from build123d import *

# Parameters (mm, degrees)
SKETCH1_R           = 3
BOSS_EXTRUDE1_DEPTH = 75
SKETCH2_R           = 5.8
BOSS_EXTRUDE2_DEPTH = 4.3
FILLET1_R           = 1


with BuildPart() as part:
    # Sketch1 → Boss-Extrude1 (new body)
    with BuildSketch(Plane(origin=(0, 0, 0), x_dir=(1, 0, 0), z_dir=(0, 1, 0))):
        with Locations(Location((0, 0, 0), (0, 0, 270))):  # turned: the seam where the file's is
            Circle(SKETCH1_R)
    extrude(amount=BOSS_EXTRUDE1_DEPTH)

    # Sketch2 → Boss-Extrude2 (add)
    with BuildSketch(Plane(origin=(0, 75, 0), x_dir=(1, 0, 0), z_dir=(0, 1, 0))):
        with Locations(Location((0, 0, 0), (0, 0, 270))):  # turned: the seam where the file's is
            Circle(SKETCH2_R)
    extrude(amount=BOSS_EXTRUDE2_DEPTH)

    # Fillet1
    fillet1_edges = [part.edges().sort_by_distance(p)[0] for p in [
        (0, 75, -5.8),
        (0, 79.3, -5.8),
    ]]
    fillet(fillet1_edges, radius=FILLET1_R)


solid = part.part
Input: part model. Units: mm. Frame: model coordinates. A direction names the side the tool comes from. Give positions to 0.01 mm unless a question says otherwise; leave off trailing zeros. Write each loop counter-clockwise with the first axis right and the second up, starting at its lowest first coordinate (ties: lowest second). Pieces come first, ordered by that corner, then holes. Notation, with made-up numbers: (74.25, 23.5) -> (132.25, 23.5) arc R28 ccw to (132.25, 45.5) -> close; hole circle Ø2 at (80.25, 63.25). An arc over 180 degrees is marked (long way). Use one line per item in the form item = value. Start each with the question number.
1) Set-up query: faces 1 (the cylindrical face through (0.255, 77.134, -5.794)), 2 (the flat face through (-3, 75, 1)). Return all of +Z, -Z, +X, -X, +Y, -Y with unobstructed straight access to the full face (end or side cutting, diameter ignored); none if empty.
2) Ray query, probe 1 along Y at (x, z) = (-3.5, 2.75); probe 2 along X at (y, z) = (73, 0); probe 3 along Y at (x, z) = (-4.75, -2.25). Return the intervals inside material, ascending. Write a range as from..to.
3) Pin query (flat end, axial travel): pin 1 (1.5 mm diameter, centred on y = 45, z = -4.5, fed in from +X); pin 2 (6 mm diameter, centred on x = -1.5, y = 26.5, fed in from +Z); pin 3 (1 mm diameter, centred on x = 2.5, z = 4.5, fed in from -Y); pin 4 (3 mm diameter, centred on x = -2.5, y = 21, fed in from +Z). Return the tip coordinate at first contact, or that it passes through.
4) Section query A-A on x = 0. Return the cut outline in (y, z), then the cut area to 3 significant figures.
5) Section query B-B on z = 0. Return the cut outline in (x, y), then the cut area to 3 significant figures.
6) Section query C-C on y = 30.5. Return the cut outline in (x, z), then the cut area to 3 significant figures.
Outcome:
q1.face_1 = +Y, -Y
q1.face_2 = -Y
q2.probe_1 = 75..79.3
q2.probe_2 = -3..3
q2.probe_3 = 75.11..79.19
q3.pin_1 = through
q3.pin_2 = 3
q3.pin_3 = 75
q3.pin_4 = 2.83
q4.outline = (0, -3) -> (75, -3) -> (75, -4.8) arc R1 ccw to (76, -5.8) -> (78.3, -5.8) arc R1 ccw to (79.3, -4.8) -> (79.3, 4.8) arc R1 ccw to (78.3, 5.8) -> (76, 5.8) arc R1 ccw to (75, 4.8) -> (75, 3) -> (0, 3) -> close
q4.area = 499 mm^2
q5.outline = (-5.8, 76) arc R1 ccw to (-4.8, 75) -> (-3, 75) -> (-3, 0) -> (3, 0) -> (3, 75) -> (4.8, 75) arc R1 ccw to (5.8, 76) -> (5.8, 78.3) arc R1 ccw to (4.8, 79.3) -> (-4.8, 79.3) arc R1 ccw to (-5.8, 78.3) -> close
q5.area = 499 mm^2
q6.outline = circle Ø6 at (0, 0)
q6.area = 28.3 mm^2
